from build123d import *

# Parameters (mm, degrees)
ESQUISSE1_W             = 60
ESQUISSE1_H             = 6
BOSS_EXTRU_1_DEPTH      = 60
ESQUISSE2_R             = 1.25
ENL_V_MAT_EXTRU_1_DEPTH = 15
ESQUISSE3_R             = 1.25
ENL_V_MAT_EXTRU_2_DEPTH = 15
ESQUISSE4_W             = 10
ESQUISSE4_H             = 11
ENL_V_MAT_EXTRU_3_DEPTH = 3
ENL_V_MAT_EXTRU_4_DEPTH = 52
CHANFREIN1_SIZE2        = 6.433520762
CHANFREIN1_SIZE         = 3


with BuildPart() as part:
    # Esquisse1 → Boss.-Extru.1 (new body)
    with BuildSketch(Plane.XY):
        with Locations((30, 3)):
            Rectangle(ESQUISSE1_W, ESQUISSE1_H)
    extrude(amount=BOSS_EXTRU_1_DEPTH)

    # Esquisse2 → Enlèv. mat.-Extru.1 (cut)
    with BuildSketch(Plane(origin=(0, 0, 0), x_dir=(-1, 0, 0), z_dir=(0, 0, -1))):
        with Locations((-54, 3)):
            Circle(ESQUISSE2_R)
        with Locations((-5.75, 3)):
            Circle(ESQUISSE2_R)
    extrude(amount=-ENL_V_MAT_EXTRU_1_DEPTH, mode=Mode.SUBTRACT)

    # Esquisse3 → Enlèv. mat.-Extru.2 (cut)
    with BuildSketch(Plane(origin=(0, 6, 0), x_dir=(1, 0, 0), z_dir=(0, 1, 0))):
        with Locations(Location((30, -37.5, 0), (0, 0, 270))):
            Circle(ESQUISSE3_R)
    extrude(amount=-ENL_V_MAT_EXTRU_2_DEPTH, mode=Mode.SUBTRACT)

    # Esquisse4 → Enlèv. mat.-Extru.3 (cut)
    with BuildSketch(Plane(origin=(0, 6, 0), x_dir=(1, 0, 0), z_dir=(0, 1, 0))):
        Polygon((0, -16), (9, -16), (9, 0), (51, 0), (51, -16), (60, -16), (60, -60), (0, -60), align=None)
        with Locations((30, -37.5)):
            Rectangle(ESQUISSE4_W, ESQUISSE4_H, mode=Mode.SUBTRACT)
    extrude(amount=-ENL_V_MAT_EXTRU_3_DEPTH, mode=Mode.SUBTRACT)

    # Esquisse5 → Enlèv. mat.-Extru.4 (cut)
    with BuildSketch(Plane(origin=(0, 3, 0), x_dir=(1, 0, 0), z_dir=(0, 1, 0))):
        Polygon((60, -16), (35, -32), (35, -43), (25, -43), (25, -32), (0, -16), (-21.594855386, -85.475485762), (75.414479662, -69.930764824), align=None)
    extrude(amount=-ENL_V_MAT_EXTRU_4_DEPTH, mode=Mode.SUBTRACT)

    # Chanfrein1
    chanfrein1_edges = [part.edges().sort_by_distance(p)[0] for p in [
        (30, 3, 32),
    ]]
    chanfrein1_side = [part.faces().sort_by_distance(p)[0] for p in [
        (30, 3.06, 32),
    ]]
    chamfer(chanfrein1_edges, length=CHANFREIN1_SIZE - 0.0001, length2=CHANFREIN1_SIZE2 - 0.0001, reference=chanfrein1_side[0])  # a hair under: the kernel refuses the full size


solid = part.part
CAD build for the part. Positions are in the model's coordinates, mm. A direction names the side the tool comes from. Give positions to 0.01 mm unless a question says otherwise; leave off trailing zeros. Order: outer loops, then holes, each group sorted by start corner. A loop starts at its lowest first (then second) coordinate and runs counter-clockwise, first axis right, second up. Notation, with made-up numbers: (13, 58) - (53, 58) arc R13 cw to (53, 75) - close; hole circle Ø6 at (-12, 52.5). An arc over 180 degrees is marked (long way). Write each question's results on one line, items separated by ' | '.
1. Pin check, flat tips, straight feed: pin 1 (1.2 mm diameter, centred on x = 5.5, y = 3.5, fed in from -Z); pin 2 (1.5 mm diameter, centred on y = 2, z = 20.5, fed in from +X); pin 3 (2 mm diameter, centred on x = 16.5, z = 26.5, fed in from +Y). Stop position of each tip, or through.
Calculated:
pin 1: stops at z = 15 | pin 2: stops at x = 54.14 | pin 3: stops at y = 3.71
2. Pull direction Z, two halves, no side cores. Call faces 1 (the face through (30.05, 3.04, 36.25)), 2 (the face through (30, 2, 0)), 3 (the face through (60, 3, 8)): released by +Z, released by -Z, zero draft, split by the parting line, or undercut.
Calculated:
face 1: undercut | face 2: released by -Z | face 3: zero draft
3. 3-axis set-ups, long thin cutter, end or side, ignore diameter. For faces 4 (the face through (51, 5, 8)), 5 (the face through (54, 3, 15)), 6 (the face through (25, 3, 38)): which of +Z, -Z, +X, -X, +Y, -Y reach the whole face in a straight line?
Calculated:
face 4: +Z, -Z, +Y | face 5: -Z | face 6: +Z, -X, +Y, -Y
4. Probe L1, parallel to X at y = 3.7, z = 14.5; L2, parallel to Y at x = 5.75, z = 11.75; L3, parallel to X at y = 4.05, z = 6. List the from-to ranges inside material, lowest first. Write a range as from..to.
Calculated:
L1: x = 0..4.71, 6.79..9, 51..52.96, 55.04..60 | L2: y = 0..1.75, 4.25..6 | L3: x = 0..5.07, 6.43..9, 51..53.32, 54.68..60
5. Saw through at D-D on x = 5.75. List the corners of the cut face in (y, z).
Calculated:
outline: (0, 0) - (1.75, 0) - (1.75, 15) - (4.25, 15) - (4.25, 0) - (6, 0) - (6, 16) - (3, 16) - (3, 19.68) - (0, 19.68) - close
6. Saw through at C-C on z = 37.5. List the corners of the cut face in (x, y), and give its area (3 significant figures).
Calculated:
outline: (25, 0) - (28.75, 0) - (28.75, 6) - (25, 6) - close; (31.25, 0) - (35, 0) - (35, 6) - (31.25, 6) - close | area: 45.0 mm2
7. Saw through at A-A on y = 0.85. List the corners of the cut face in (x, z), and give its area (3 significant figures).
Calculated:
outline: (0, 0) - (60, 0) - (60, 16) - (35, 32) - (35, 43) - (25, 43) - (25, 32) - (0, 16) - close; hole circle Ø2.5 at (30, 37.5) | area: 1,630 mm2
